```python
from build123d import *

# Parameters (mm, degrees)
BOSS_EXTRUDE1_DEPTH      = 0.8
BOSS_EXTRUDE1_DEPTH_BACK = 0.8
FILLET1_R                = 1


with BuildPart() as part:
    # Sketch2 → Boss-Extrude1 (new body, two sides)
    with BuildSketch(Plane(origin=(23.824934682, 0, 0), x_dir=(0, 0, -1), z_dir=(1, 0, 0))) as boss_extrude1_sk:
        with BuildLine():
            Line((-65.407740568, 112.017340514), (7.473597983, 112.017340514))
            Line((7.473597983, 112.017340514), (7.473597983, 57.27523093))
            Line((7.473597983, 57.27523093), (-11.887740568, 57.27523093))
            Line((-11.887740568, 57.27523093), (-11.887740568, 51.84523093))
            Line((-11.887740568, 51.84523093), (-12.387740568, 51.34523093))
            Line((-12.387740568, 51.34523093), (-30.007740568, 51.34523093))
            Line((-30.007740568, 51.34523093), (-30.507740568, 51.84523093))
            Line((-30.507740568, 51.84523093), (-30.507740568, 57.27523093))
            ThreePointArc((-30.507740568, 57.27523093), (-31.387740568, 58.15523093), (-32.267740568, 57.27523093))
            Line((-32.267740568, 57.27523093), (-32.267740568, 51.84523093))
            Line((-32.267740568, 51.84523093), (-32.767740568, 51.34523093))
            Line((-32.767740568, 51.34523093), (-41.992740568, 51.34523093))
            Line((-41.992740568, 51.34523093), (-42.492740568, 51.84523093))
            Line((-42.492740568, 51.84523093), (-42.492740568, 57.27523093))
            ThreePointArc((-42.492740568, 57.27523093), (-43.647740568, 58.43023093), (-44.802740568, 57.27523093))
            Line((-44.802740568, 57.27523093), (-44.802740568, 51.84523093))
            Line((-44.802740568, 51.84523093), (-45.302740568, 51.34523093))
            Line((-45.302740568, 51.34523093), (-63.102740568, 51.34523093))
            Line((-63.102740568, 51.34523093), (-63.602740568, 51.84523093))
            Line((-63.602740568, 51.84523093), (-63.602740568, 57.27523093))
            Line((-63.602740568, 57.27523093), (-65.407740568, 57.27523093))
            Line((-65.407740568, 57.27523093), (-65.407740568, 112.017340514))
        make_face()
    extrude(amount=BOSS_EXTRUDE1_DEPTH)
    extrude(boss_extrude1_sk.sketch, amount=-BOSS_EXTRUDE1_DEPTH_BACK)

    # Fillet1
    fillet1_edges = [part.edges().sort_by_distance(p)[0] for p in [
        (23.824934682, 112.017340514, 65.407740568),
        (23.824934682, 112.017340514, -7.473597983),
        (23.824934682, 57.27523093, -7.473597983),
        (23.824934682, 57.27523093, 65.407740568),
    ]]
    fillet(fillet1_edges, radius=FILLET1_R)


solid = part.part
```
Source: CAD feature listing. Evaluate the final solid. Frame: model axes, mm. A direction names the side the tool comes from. Coordinates: 2 decimals unless noted, no trailing zeros. Write each loop counter-clockwise with the first axis right and the second up, starting at its lowest first coordinate (ties: lowest second). Pieces come first, ordered by that corner, then holes. Notation, with made-up numbers: (47.25, -13) - (73.25, -13) arc R20 cw to (73.25, 14) - close; hole circle Ø9 at (-15, -30.75). An arc over 180 degrees is marked (long way). Answer as a JSON object with one key per item and string values.
Q1. Section query A-A, the plane x = 23.7. Output: boundary loops of the cut face in (y, z) (3 decimals), plus the area to 3 significant figures.
Ans:
{"outline": "(51.345, 12.388) - (51.845, 11.888) - (57.275, 11.888) - (57.275, -6.474) arc R1 ccw to (58.275, -7.474) - (111.017, -7.474) arc R1 ccw to (112.017, -6.474) - (112.017, 64.408) arc R1 ccw to (111.017, 65.408) - (58.275, 65.408) arc R1 ccw to (57.275, 64.408) - (57.275, 63.603) - (51.845, 63.603) - (51.345, 63.103) - (51.345, 45.303) - (51.845, 44.803) - (57.275, 44.803) arc R1.155 cw to (57.275, 42.493) - (51.845, 42.493) - (51.345, 41.993) - (51.345, 32.768) - (51.845, 32.268) - (57.275, 32.268) arc R0.88 cw to (57.275, 30.508) - (51.845, 30.508) - (51.345, 30.008) - close", "area": "4,270 mm2"}
Q2. First-contact query: pin 1 Ø0.6 at (x, z) = (23.5, 64) entering from -Y; pin 2 Ø0.8 at (x, y) = (24, 53.5) entering from +Z; pin 3 Ø0.5 at (x, y) = (23.5, 54.5) entering from -Z. Flat tips, straight axial feed; report the tip coordinate or a pass-through.
Ans:
{"pin 1": "stops at y = 57.28", "pin 2": "stops at z = 63.6", "pin 3": "stops at z = 11.89"}
Q3. Section query B-B, the plane z = 44. Output: boundary loops of the cut face in (x, y), plus the area to 3 significant figures.
Ans:
{"outline": "(23.02, 58.38) - (24.62, 58.38) - (24.62, 112.02) - (23.02, 112.02) - close", "area": "85.8 mm2"}
Q4. Material intervals for line 1 (Z direction, x = 23.15, y = 55.5); line 2 (Y direction, x = 23.95, z = 9.5); line 3 (Y direction, x = 23.1, z = 43), sorted ascending. Write a range as [from, to].
Ans:
{"line 1": "z = [11.89, 30.51], [32.27, 42.49], [44.8, 63.6]", "line 2": "y = [57.28, 112.02]", "line 3": "y = [58.23, 112.02]"}
Q5. Set-up query: faces 1 (the flat face through (24, 84, 65.408)), 2 (the flat face through (24, 55, 44.803)), 3 (the flat face through (24, 57.275, 3)). Return all of +Z, -Z, +X, -X, +Y, -Y with unobstructed straight access to the full face (end or side cutting, diameter ignored); none if empty.
Ans:
{"face 1": "+Z, +X, -X, +Y, -Y", "face 2": "+X, -X, -Y", "face 3": "-Z, +X, -X, -Y"}
Q6. Draft query along Z for faces 4 (the flat face through (24, 85, -7.474)), 5 (the flat face through (24, 55, 63.603)), 6 (the cylindrical face through (23.836, 58.155, 31.368)). Return one class per face: released by +Z, released by -Z, zero draft, split by the parting line, or undercut.
Ans:
{"face 4": "released by -Z", "face 5": "released by +Z", "face 6": "undercut"}
